Input: part model. Units: mm. Frame: model coordinates. Face numbers are marked on the shaded views. A direction names the side the tool comes from. Round coordinates to 2 decimals unless told otherwise and drop trailing zeros. Order: outer loops, then holes, each group sorted by start corner. A loop starts at its lowest first (then second) coordinate and runs counter-clockwise, first axis right, second up. Notation, with made-up numbers: (6.5, -40) -> (53.5, -40) arc R31 ccw to (53.5, -14) -> close; hole circle Ø7 at (3, 59.5). An arc over 180 degrees is marked (long way). Answer as CSV lines item,"result". Start each with the question number.
1) First-contact query: P1, Ø2, axis at x = -7.5, z = -16.5, coming from the -Y side; P2, Ø3, axis at x = -3.5, y = 2.5, coming from the -Z side. Flat tips, straight axial feed; report the tip coordinate or a pass-through.
2) Mould query, pull axis X, two halves, no side actions, for the marked faces 3 and 4. Classes: +X half, -X half, draft (parallel to the pull), parting line (faces both ways), or undercut.
3) Section query B-B, the plane z = -14. State how many separate pieces and enclosed holes the cut face has, and give its area (3 significant figures).
4) Line query: L1, parallel to Z at x = 0, y = 7.5; L2, parallel to X at y = 4.5, z = -79; L3, parallel to X at y = 3.5, z = -23.5. Output: solid intervals per line, ascending.
5) Access query for the marked faces 1 and 2. Directions: +Z, -Z, +X, -X, +Y, -Y. A direction counts if a zero-diameter tool reaches every point of the face in a straight line with its end or side. Return the directions, or none.
6) Section query A-A, the plane x = 33. Output: boundary loops of the cut face in (y, z).
```python
from build123d import *

# Parameters (mm, degrees)
SKETCH1_W             = 100
SKETCH1_H             = 200
BOSS_EXTRUDE1_DEPTH   = 15
SKETCH4_W             = 20
SKETCH4_H             = 30
SKETCH4_W_2           = 7
SKETCH4_H_2           = 104
CUT_EXTRUDE2_DEPTH    = 5
FILLET3_R             = 10
FILLET4_R             = 5
SKETCH8_W             = 20
SKETCH8_H             = 180
SKETCH8_W_2           = 3
SKETCH8_H_2           = 100
SKETCH8_H_3           = 6
CUT_EXTRUDE3_DEPTH    = 15
FILLET5_R             = 5
FILLET8_R             = 2.5
FILLET7_R             = 2.5
FILLET10_R            = 1.5
F_3_0MM_DOWEL_HOLE1_D = 3
F_3_0MM_DOWEL_HOLE2_D = 3


with BuildPart() as part:
    # Sketch1 → Boss-Extrude1 (new body)
    with BuildSketch(Plane(origin=(0, 0, 0), x_dir=(1, 0, 0), z_dir=(0, 1, 0))):
        Rectangle(SKETCH1_W, SKETCH1_H)
    extrude(amount=BOSS_EXTRUDE1_DEPTH)

    # Sketch4 → Cut-Extrude2 (cut)
    with BuildSketch(Plane.XZ):
        with Locations((0, 85)):
            Rectangle(SKETCH4_W, SKETCH4_H)
        with Locations((0, -85)):
            Rectangle(SKETCH4_W, SKETCH4_H)
        with Locations((-6.5, 0)):
            Rectangle(SKETCH4_W_2, SKETCH4_H_2)
        with Locations((6.5, 0)):
            Rectangle(SKETCH4_W_2, SKETCH4_H_2)
    extrude(amount=-CUT_EXTRUDE2_DEPTH, mode=Mode.SUBTRACT)

    # Fillet3
    fillet3_edges = [part.edges().sort_by_distance(p)[0] for p in [
        (50, 7.5, 100),
        (-50, 7.5, 100),
        (-50, 7.5, -100),
        (50, 7.5, -100),
    ]]
    fillet(fillet3_edges, radius=FILLET3_R)

    # Fillet4
    fillet4_edges = [part.edges().sort_by_distance(p)[0] for p in [
        (0, 15, -100),
        (50, 15, 0),
        (-50, 15, 0),
        (0, 15, 100),
        (47.071067812, 15, 97.071067812),
        (-47.071067812, 15, 97.071067812),
        (-47.071067812, 15, -97.071067812),
        (47.071067812, 15, -97.071067812),
    ]]
    fillet(fillet4_edges, radius=FILLET4_R)

    # Sketch8 → Cut-Extrude3 (cut)
    with BuildSketch(Plane.XZ):
        with Locations((30, 0)):
            Rectangle(SKETCH8_W, SKETCH8_H)
        with Locations((-30, 0)):
            Rectangle(SKETCH8_W, SKETCH8_H)
        with Locations((-6.5, 0)):
            Rectangle(SKETCH8_W_2, SKETCH8_H_2)
        with Locations((6.5, 0)):
            Rectangle(SKETCH8_W_2, SKETCH8_H_2)
        with Locations((0, 61)):
            Rectangle(SKETCH8_W, SKETCH8_H_3)
    extrude(amount=-CUT_EXTRUDE3_DEPTH, mode=Mode.SUBTRACT)

    # Fillet5
    fillet5_edges = [part.edges().sort_by_distance(p)[0] for p in [
        (20, 7.5, -90),
        (20, 7.5, 90),
        (40, 7.5, 90),
        (40, 7.5, -90),
        (-40, 7.5, -90),
        (-40, 7.5, 90),
        (-20, 7.5, 90),
        (-20, 7.5, -90),
    ]]
    fillet(fillet5_edges, radius=FILLET5_R)

    # Fillet8
    fillet8_edges = [part.edges().sort_by_distance(p)[0] for p in [
        (-10, 7.5, 58),
        (-10, 7.5, 64),
        (10, 7.5, 64),
        (10, 7.5, 58),
    ]]
    fillet(fillet8_edges, radius=FILLET8_R)

    # Fillet7
    fillet7_edges = [part.edges().sort_by_distance(p)[0] for p in [
        (-30, 15, -90),
        (-40, 15, 0),
        (-20, 15, 0),
        (30, 15, -90),
        (20, 15, 0),
        (40, 15, 0),
        (-30, 15, 90),
        (30, 15, 90),
        (-38.535533906, 15, -88.535533906),
        (-21.464466094, 15, -88.535533906),
        (21.464466094, 15, -88.535533906),
        (38.535533906, 15, -88.535533906),
        (-21.464466094, 15, 88.535533906),
        (-38.535533906, 15, 88.535533906),
        (21.464466094, 15, 88.535533906),
        (38.535533906, 15, 88.535533906),
        (0, 15, 64),
        (10, 15, 61),
        (0, 15, 58),
        (-10, 15, 61),
        (9.267766953, 15, 63.267766953),
        (9.267766953, 15, 58.732233047),
        (-9.267766953, 15, 58.732233047),
        (-9.267766953, 15, 63.267766953),
    ]]
    fillet(fillet7_edges, radius=FILLET7_R)

    # Fillet10
    fillet10_edges = [part.edges().sort_by_distance(p)[0] for p in [
        (8, 10, -50),
        (5, 10, -50),
        (-5, 10, -50),
        (-8, 10, -50),
        (5, 10, 50),
        (8, 10, 50),
        (-8, 10, 50),
        (-5, 10, 50),
    ]]
    fillet(fillet10_edges, radius=FILLET10_R - 0.0001)  # a hair under: the kernel refuses the full size

    # Ø3.0mm Dowel Hole1 (through all)
    with Locations(Plane(origin=(0, 5, 0), x_dir=(-1, 0, 0), z_dir=(0, -1, 0))):
        with Locations((0, 77.5), (0, 92.5)):
            Hole(F_3_0MM_DOWEL_HOLE1_D / 2)

    # Ø3.0mm Dowel Hole2 (through all)
    with Locations(Plane(origin=(0, 5, 0), x_dir=(-1, 0, 0), z_dir=(0, -1, 0))):
        with Locations((0, -92.5), (0, -77.5)):
            Hole(F_3_0MM_DOWEL_HOLE2_D / 2)


solid = part.part
```
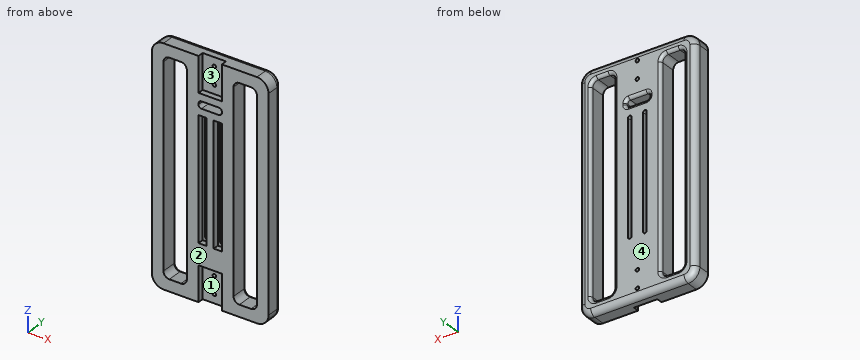
Findings:
1,P1,"stops at y = 5"
1,P2,"stops at z = -70"
2,face 3,"undercut"
2,face 4,"draft"
3,separate pieces,"5"
3,enclosed holes,"0"
3,area,"754 mm^2"
4,L1,"z = -100 to -94, -91 to -79, -76 to 58, 64 to 76, 79 to 91, 94 to 100"
4,L2,"x = -50 to -40, -20 to -10, 10 to 20, 40 to 50"
4,L3,"x = -50 to -40, -20 to -10, -3 to 3, 10 to 20, 40 to 50"
5,face 1,"-Z, -Y"
5,face 2,"+Z, -Z, +X, -X, -Y"
6,outline,"(0, -100) -> (10, -100) arc R5 ccw to (15, -95) -> (15, -92.5) arc R2.5 ccw to (12.5, -90) -> (0, -90) -> close; (0, 90) -> (12.5, 90) arc R2.5 ccw to (15, 92.5) -> (15, 95) arc R5 ccw to (10, 100) -> (0, 100) -> close"
